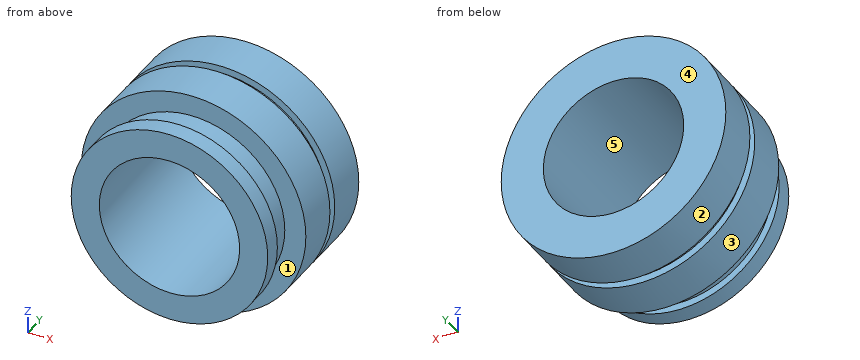
Autodesk Fusion 360 part; units mm, degrees
sketch "Sketch1" plane through (0, 0, 0) normal (0, 0, 1) x (1, 0, 0)
  line L0 (2, 0) -> (2.8, 0)
  line L1 (2.8, 0) -> (2.8, 0.5)
  line L2 (2.8, 0.5) -> (2.6, 0.5)
  line L3 (2.6, 0.5) -> (2.6, 1.25)
  line L4 (2.6, 1.25) -> (3.2, 1.25)
  line L5 (3.2, 4) -> (2, 4)
  line L6 (2, 4) -> (2, 0)
  line L7 (3.2, 2.75) -> (3, 2.75)
  line L8 (3, 2.75) -> (3, 2.5)
  line L9 (3, 2.5) -> (3.2, 2.5)
  line L10 (3.2, 1.25) -> (3.2, 2.5)
  line L11 (3.2, 2.75) -> (3.2, 4)
  dimension "d1" = 4
  dimension "d6" = 2
  dimension "d7" = 2.8
  dimension "d8" = 3.2
  dimension "d9" = 2.75
  dimension "d10" = 0.5
  dimension "d11" = 0.25
  dimension "d12" = 0.2
  dimension "d13" = 0.2
revolve "Revolve1" add sketch "Sketch1" angle 360 about axis through (0, 1.75, 0) along (0, 1, 0)
thread "Thread1"
equation "d7 = ( 5.6 / 2 ) * 1 mm"
equation "d8 = ( 6.4 / 2 ) * 1 mm"
Geometry check sheet. Reference: the model listing, model coordinates, mm. Face numbers are marked on the shaded views. A direction names the side the tool comes from. Give positions to 0.01 mm unless a question says otherwise; leave off trailing zeros. Order: outer loops, then holes, each group sorted by start corner. A loop starts at its lowest first (then second) coordinate and runs counter-clockwise, first axis right, second up.
1. Scan lines: line 1 (Z direction, x = 0, y = 1); line 2 (Y direction, x = -0.5, z = 3); line 3 (X direction, y = 1.75, z = 0). Record each from-to range of solid material in increasing order.
Completed:
line 1: z = -2.6 to -2, 2 to 2.6
line 2: y = 1.25 to 2.5, 2.75 to 4
line 3: x = -3.2 to -2, 2 to 3.2
2. Access from +Z, -Z, +X, -X, +Y, -Y to the whole of each face (thin tool, end or side, straight path). Record for the marked faces 1 and 2.
Completed:
face 1: none
face 2: +Y, -Y
3. Sectioned sample at B-B (z = 0). Record the boundary of the cut face in (x, y).
Completed:
outline: (-3.2, 1.25) - (-2.6, 1.25) - (-2.6, 0.5) - (-2.8, 0.5) - (-2.8, 0) - (-2, 0) - (-2, 4) - (-3.2, 4) - (-3.2, 2.75) - (-3, 2.75) - (-3, 2.5) - (-3.2, 2.5) - close; (2, 0) - (2.8, 0) - (2.8, 0.5) - (2.6, 0.5) - (2.6, 1.25) - (3.2, 1.25) - (3.2, 2.5) - (3, 2.5) - (3, 2.75) - (3.2, 2.75) - (3.2, 4) - (2, 4) - close
4. Sectioned sample at C-C (y = 0.3). Record the boundary of the cut face in (x, z).
Completed:
outline: circle Ø5.6 at (0, 0); hole circle Ø4 at (0, 0)
5. Draft check along Z on the marked faces 3, 4 and 5. Enter one of: pulls with the +Z half, pulls with the -Z half, needs draft (parallel to the pull), parting line crosses it, or undercut.
Completed:
face 3: parting line crosses it
face 4: needs draft
face 5: undercut
6. Sectioned sample at D-D (x = 2.25). Record the boundary of the cut face in (y, z).
Completed:
outline: (0, -1.67) - (0.5, -1.67) - (0.5, -1.3) - (1.25, -1.3) - (1.25, -2.28) - (2.5, -2.28) - (2.5, -1.98) - (2.75, -1.98) - (2.75, -2.28) - (4, -2.28) - (4, 2.28) - (2.75, 2.28) - (2.75, 1.98) - (2.5, 1.98) - (2.5, 2.28) - (1.25, 2.28) - (1.25, 1.3) - (0.5, 1.3) - (0.5, 1.67) - (0, 1.67) - close
7. Sectioned sample at A-A (x = 0). Record the boundary of the cut face in (y, z).
Completed:
outline: (0, -2.8) - (0.5, -2.8) - (0.5, -2.6) - (1.25, -2.6) - (1.25, -3.2) - (2.5, -3.2) - (2.5, -3) - (2.75, -3) - (2.75, -3.2) - (4, -3.2) - (4, -2) - (0, -2) - close; (0, 2) - (4, 2) - (4, 3.2) - (2.75, 3.2) - (2.75, 3) - (2.5, 3) - (2.5, 3.2) - (1.25, 3.2) - (1.25, 2.6) - (0.5, 2.6) - (0.5, 2.8) - (0, 2.8) - close
